Autodesk Inventor part; units mm, degrees
ref_plane "Work Plane1" through (76.2, 0, 0) normal (1, 0, 0) x (0, 1, 0)
ref_plane "XZ Plane" through (0, 0, 0) normal (0, 1, 0) x (-1, 0, 0)
ref_plane "XY Plane" through (0, 0, 0) normal (0, 0, 1) x (1, 0, 0)
sketch "Sketch2" plane through (0, 0, 0) normal (0, 0, 1) x (1, 0, 0)
  circle A0 centre (0, 0) radius 9.525
  dimension "d3" = 19.05
extrude "Extrusion2" add sketch "Sketch2" against normal blind 1517.65
ref_plane "Work Plane1" through (76.2, 0, 0) normal (1, 0, 0) x (0, 1, 0)
sketch "Sketch9" plane through (76.2, 0, 0) normal (1, 0, 0) x (0, 1, 0)
  line L0 (-9.525, -1517.65) -> (9.525, -1517.65)
  circle A0 centre (0, -1593.85) radius 9.525
  line L1 (0, -1517.65) -> (0, -1593.85) construction
  point P0 (0, 0)
  dimension "d17" = 19.05
  dimension "d18" = 76.2
extrude "Extrusion4" add sketch "Sketch9" along normal blind 1365.25
sketch "Sketch11" plane through (0, 0, -1517.65) normal (0, 0, -1) x (-1, 0, 0)
  circle A0 centre (0, 0) radius 9.525
sketch "Sketch12" plane through (0, 0, 0) normal (0, 1, 0) x (-1, 0, 0)
  line L0 (-76.2, -1603.375) -> (-76.2, -1584.325)
  line L1 (-9.525, -1517.65) -> (9.525, -1517.65)
  arc A0 (-76.2, -1593.85) -> (0, -1517.65) centre (-76.2, -1517.65) ccw
  point P0 (0, 0)
  dimension "d21" = 76.2
sweep "Sweep2" add profiles "Sketch11" path "Sketch12" path curves A0
equation "\"d3\" = tubeD"
equation "\"d17\" = tubeD"
equation "\"d18\" = tubeTurnR"
equation "\"d21\" = tubeTurnR"
equation "\"d4\" = tubeTurnR"
equation "\"wallThick\" = 44.45"
equation "\"roomWidth\" = 3048"
equation "\"roomDepth\" = 3657.6"
equation "\"roomHeight\" = 2438.4"
equation "\"doorWidth\" = 895.35"
equation "\"doorHeight\" = 2108.2"
equation "\"doorX\" = 774.7"
equation "\"doorY\" = 88.9"
equation "\"doorLip\" = 76.2"
equation "\"doorThick\" = 57.15"
equation "\"tubeTurnR\" = 76.2"
equation "\"tubeD\" = 19.05"
properties part number "left_tube_0"
Work out the finished part from the listing and answer in its coordinate system (mm). Round coordinates to 2 decimals unless told otherwise and drop trailing zeros. Loops run counter-clockwise (first coordinate to the right, second up) from the corner with the lowest first, then second, coordinate; pieces in that order, holes last. Notation, with made-up numbers: M -1.5,38 L 49.5,38 A9 ccw 49.5,47 Z; hole C 56,-37 d1. An arc over 180 degrees is marked long. Use CSV: the item, a comma, the result in double quotes.
Q1. Section A-A, the plane y = 0 is taken. Determine the outline of the cut face in (x, z) (3 decimals).
Determined:
outline,"M -9.525,-1517.65 A85.725 ccw 76.2,-1603.375 L 1441.45,-1603.375 L 1441.45,-1584.325 L 76.2,-1584.325 A66.675 cw 9.525,-1517.65 L 9.525,0 L -9.525,0 Z"
Q2. Each of these flat-tipped pins is pushed along its axis until it touches: pin 1 (2 mm diameter, centred on y = -3.5, z = -606, fed in from +X); pin 2 (8 mm diameter, centred on x = 1098, y = 1.5, fed in from +Z) (3 decimals); pin 3 (2 mm diameter, centred on y = -5, z = -1089.5, fed in from +X). Where does it stop, or does it pass through?
Determined:
pin 1,"x = 9.19"
pin 2,"z = -1584.325"
pin 3,"x = 8.64"
Q3. Section B-B, the plane z = -1270 is taken. Determine the outline of the cut face in (x, y) (3 decimals).
Determined:
outline,"C 0,0 d19.05"
Q4. Section C-C, the plane x = 895 is taken. Determine the outline of the cut face in (y, z) (3 decimals).
Determined:
outline,"C 0,-1593.85 d19.05"
Q5. Consider L1, parallel to Z at x = 903, y = -2; L2, parallel to X at y = 2.25, z = -983.5; L3, parallel to Z at x = 594, y = 1.5. Determine where each line is inside the solid, lowest interval first.
Determined:
L1,"-1603.16 to -1584.54"
L2,"-9.26 to 9.26"
L3,"-1603.26 to -1584.44"
